Study the drawing (mm; zero at the part's minimum x, y, z) and answer. A direction names the side the tool comes from. Round coordinates to 2 decimals unless told otherwise and drop trailing zeros. Loops run counter-clockwise (first coordinate to the right, second up) from the corner with the lowest first, then second, coordinate; pieces in that order, holes last. Notation, with made-up numbers: M 34,81 L 84,81 A9 ccw 84,85 Z; hole C 4,53 d8. An arc over 180 degrees is marked long. Write each question's results on one line, items separated by ' | '.
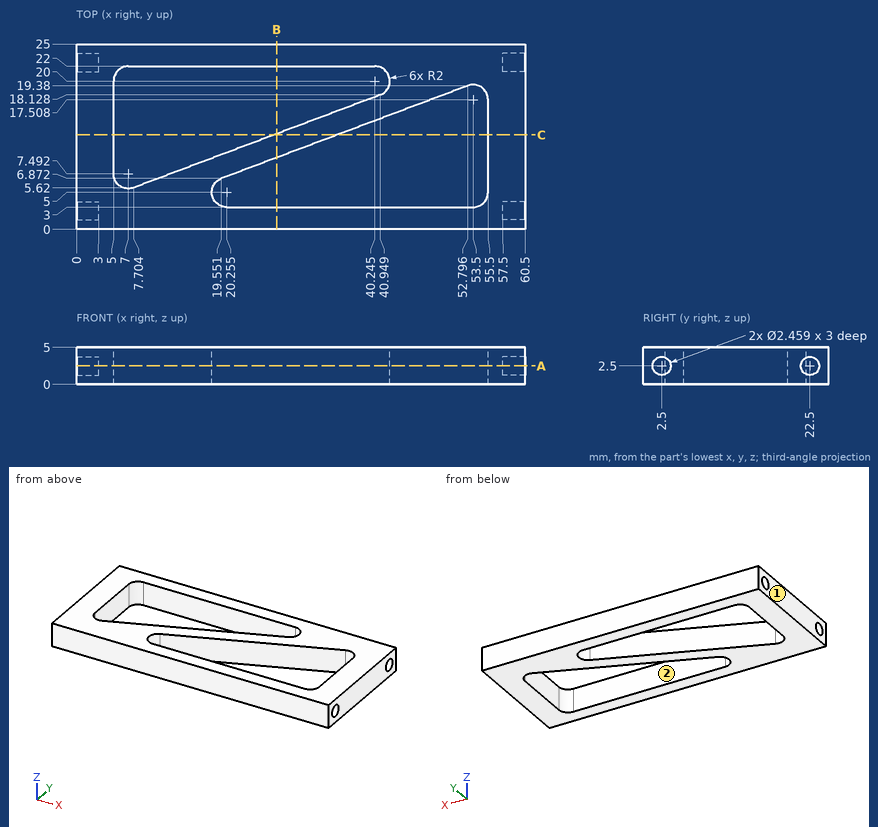
Item 1: The part is cut by section C-C (y = 12.75). Determine the outline of the cut face in (x, z) (1 decimal), plus the area to 3 significant figures.
Outcome:
outline: M 0,0 L 5,0 L 5,5 L 0,5 Z; M 26.7,0 L 35.2,0 L 35.2,5 L 26.7,5 Z; M 55.5,0 L 60.5,0 L 60.5,5 L 55.5,5 Z | area: 92.6 mm2
Item 2: The part is cut by section A-A (z = 2.5). State how many separate pieces and enclosed holes the cut face has, plus the area to 3 significant figures.
Outcome:
separate pieces: 1 | enclosed holes: 2 | area: 717 mm2
Item 3: For the marked faces 1 and 2, determine the directions among +Z, -Z, +X, -X, +Y, -Y from which every point of the face is accessible in a straight line to the end or side of a thin tool.
Outcome:
face 1: +Z, -Z, -X, +Y, -Y | face 2: +Z, -Z
Item 4: The part is cut by section B-B (x = 27). Determine the outline of the cut face in (y, z) (1 decimal).
Outcome:
outline: M 0,0 L 3,0 L 3,5 L 0,5 Z; M 9.7,0 L 12.9,0 L 12.9,5 L 9.7,5 Z; M 22,0 L 25,0 L 25,5 L 22,5 Z
Item 5: Flat-ended cylindrical pins translate along their axes: pin 1 (5 mm diameter, centred on x = 19, y = 18, fed in from +Z); pin 2 (1.2 mm diameter, centred on y = 22.5, z = 2.5, fed in from -X); pin 3 (0.7 mm diameter, centred on y = 2.5, z = 3, fed in from +X). Find the tip coordinate at first contact, or state that the pin passes through.
Outcome:
pin 1: passes through | pin 2: stops at x = 3 | pin 3: stops at x = 57.5
Item 6: Straight lines are drawn through the part: line 1 (Y direction, x = 58.25, z = 2.5); line 2 (Z direction, x = 59.35, y = 2.5); line 3 (Y direction, x = 25, z = 2.4). For each, find the intervals that lie inside material, in ascending order.
Outcome:
line 1: y = 0 to 1.27, 3.73 to 21.27, 23.73 to 25 | line 2: z = 0 to 1.27, 3.73 to 5 | line 3: y = 0 to 3, 8.92 to 12.13, 22 to 25
